```python
from build123d import *

# Parameters (mm, degrees)
F0_R     = 15.875
F1_DEPTH = 1.778
F3_R     = 0.889
F4_DEPTH = 1.016
F5_R     = 1.524
F5_W     = 3.048
F5_H     = 6.400035
F6_DEPTH = 2.22015


with BuildPart() as f1:
    # F0 (on Top) → F1 (new body)
    with BuildSketch(Plane.XY):
        Circle(F0_R)
    extrude(amount=-F1_DEPTH)

    # F3 (on face) → F4 (join)
    with BuildSketch(Plane.XY):
        with Locations((0, 13.652203)):
            Circle(F3_R)
        with Locations((-13.659894, -0.015021)):
            Circle(F3_R)
        with Locations((13.674476, -0.124876)):
            Circle(F3_R)
    extrude(amount=F4_DEPTH)

    # F5 (on face) → F6 (cut)
    with BuildSketch(Plane.XY):
        Circle(F5_R)
        with Locations((0, 5.805492)):
            Rectangle(F5_W, F5_H)
    extrude(amount=-F6_DEPTH, mode=Mode.SUBTRACT)


solid = f1.part
```
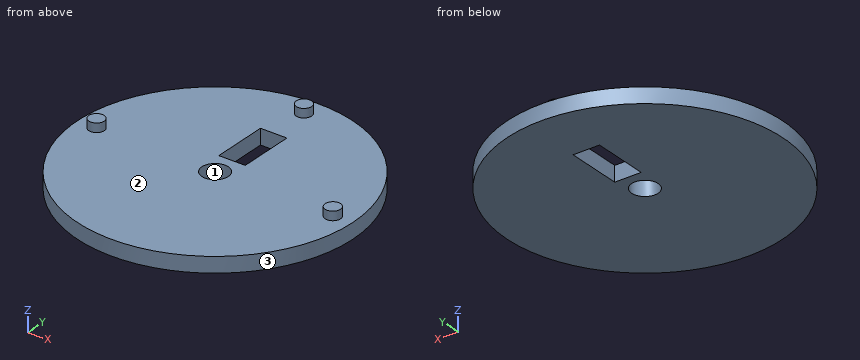
Model file for the job. Use its own axes, mm. Face numbers are marked on the shaded views. Coordinates: 2 decimals unless noted, no trailing zeros. Order: outer loops, then holes, each group sorted by start corner. A loop starts at its lowest first (then second) coordinate and runs counter-clockwise, first axis right, second up. Notation, with made-up numbers: (33.25, 77) -> (63.25, 77) arc R5 ccw to (63.25, 84) -> close; hole circle Ø7 at (-4, 1). An arc over 180 degrees is marked (long way). Return JSON: item names as keys, results as strings.
Item 1: Slice it at D-D (y = -6.5). Write the cut outline in (x, z), then the cut area to 3 significant figures.
Model answer:
{"outline": "(-14.48, -1.78) -> (14.48, -1.78) -> (14.48, 0) -> (-14.48, 0) -> close", "area": "51.5 mm²"}
Item 2: Slice it at C-C (x = -13.5). Write the cut outline in (y, z), then the cut area to 3 significant figures.
Model answer:
{"outline": "(-8.35, -1.78) -> (8.35, -1.78) -> (8.35, 0) -> (0.86, 0) -> (0.86, 1.02) -> (-0.89, 1.02) -> (-0.89, 0) -> (-8.35, 0) -> close", "area": "31.5 mm²"}
Item 3: Slice it at A-A (x = 0). Write the cut outline in (y, z) (1 decimal), then the cut area to 3 significant figures.
Model answer:
{"outline": "(-15.9, -1.8) -> (-1.5, -1.8) -> (-1.5, 0) -> (-15.9, 0) -> close; (1.5, -1.8) -> (2.6, -1.8) -> (2.6, 0) -> (1.5, 0) -> close; (9, -1.8) -> (15.9, -1.8) -> (15.9, 0) -> (14.5, 0) -> (14.5, 1) -> (12.8, 1) -> (12.8, 0) -> (9, 0) -> close", "area": "41.5 mm²"}
Item 4: Pin check, flat tips, straight feed: P1, Ø1.4, axis at x = -0.5, z = -1, coming from the -Y side (3 decimals); P2, Ø1, axis at y = 6.5, z = 0, coming from the -X side; P3, Ø1, axis at x = 1.5, z = 0, coming from the +Y side; P4, Ø0.9, axis at y = 4.5, z = -1, coming from the +X side. Stop position of each tip, or through.
Model answer:
{"P1": "stops at y = -15.875", "P2": "stops at x = -14.7", "P3": "stops at y = 15.84", "P4": "stops at x = 15.35"}
Item 5: Slice it at B-B (z = -1.3). Count the separate pieces of the cut face and the enclosed holes in it, then the cut area to 3 significant figures.
Model answer:
{"separate pieces": "1", "enclosed holes": "2", "area": "765 mm²"}
Item 6: Wall check: line 1 along Y through (x, z) = (0, -0.35) (1 decimal); line 2 along Z through (x, y) = (-6, -1); line 3 along X through (y, z) = (4, -0.35). Give the ranges that are in metal, low to high. Write a range as from..to.
Model answer:
{"line 1": "y = -15.9..-1.5, 1.5..2.6, 9..15.9", "line 2": "z = -1.78..0", "line 3": "x = -15.36..-1.52, 1.52..15.36"}
Item 7: Mould opens along Y. For the marked faces 1, 2 and 3 say: pulls with the +Y half, pulls with the -Y half, needs draft (parallel to the pull), parting line crosses it, or undercut.
Model answer:
{"face 1": "undercut", "face 2": "needs draft", "face 3": "parting line crosses it"}
